Could you check a few things on this model? Use its own coordinates, in mm. A direction names the side the tool comes from. Give positions to 0.01 mm unless a question says otherwise; leave off trailing zeros. Order: outer loops, then holes, each group sorted by start corner. A loop starts at its lowest first (then second) coordinate and runs counter-clockwise, first axis right, second up. Notation, with made-up numbers: (20, 73) - (40, 73) arc R17 cw to (40, 79) - close; hole circle Ø5 at (-18, 41.5). An arc over 180 degrees is marked (long way). Put each result on its own line as item: value.
from build123d import *

# Parameters (mm, degrees)
EXTRUDE_1_DEPTH              = 10
SKETCH_2_3_W                 = 10
SKETCH_2_3_H                 = 57
EXTRUDE_2_DEPTH              = 80
HOLE_WIZARD_M3_2_D           = 3.4
HOLE_WIZARD_M3_2_CSINK_D     = 3.65
HOLE_WIZARD_M3_2_CSINK_ANGLE = 90
CUT_EXTRUDE_1_REACH          = 102.372
HOLE_WIZARD_M3_3_D           = 3.4
HOLE_WIZARD_M3_3_CSINK_D     = 3.65
HOLE_WIZARD_M3_3_CSINK_ANGLE = 90
CHAMFER_2_SIZE               = 3
CHAMFER_3_SIZE               = 6
PATTERN_CIRCULAR_1_COUNT     = 4
SKETCH_13_R                  = 2.5
EXTRUDE_3_DEPTH              = 6
HOLE_WIZARD_M3_1_D           = 2.5
HOLE_WIZARD_M3_1_DEPTH       = 5
HOLE_WIZARD_M3_1_CSINK_D     = 3.05
HOLE_WIZARD_M3_1_CSINK_ANGLE = 90
HOLE_WIZARD_M3_1_TIP         = 0.751075774


with BuildPart() as part:
    # 草图2 → 凸台-拉伸1 (new body)
    with BuildSketch(Plane(origin=(0, 0, 0), x_dir=(1, 0, 0), z_dir=(0, 1, 0))):
        with BuildLine():
            Line((25, 28.5), (0, 28.5))
            ThreePointArc((0, 28.5), (-28.5, 0), (0, -28.5))
            Line((0, -28.5), (25, -28.5))
            Line((25, -28.5), (25, 28.5))
        make_face()
    extrude(amount=EXTRUDE_1_DEPTH)

    # 草图2<3> → 凸台-拉伸2 (add)
    with BuildSketch(Plane(origin=(0, 0, 0), x_dir=(1, 0, 0), z_dir=(0, 1, 0))):
        with Locations((30, 0)):
            Rectangle(SKETCH_2_3_W, SKETCH_2_3_H)
    extrude(amount=EXTRUDE_2_DEPTH)

    # M3 间隙孔2 (through all)
    with Locations(Plane(origin=(0, 10, 0), x_dir=(1, 0, 0), z_dir=(0, 1, 0))):
        with Locations((-13.435028843, 13.435028843), (13.435028843, 13.435028843), (13.435028843, -13.435028843), (-13.435028843, -13.435028843)):
            CounterSinkHole(HOLE_WIZARD_M3_2_D / 2, HOLE_WIZARD_M3_2_CSINK_D / 2, counter_sink_angle=HOLE_WIZARD_M3_2_CSINK_ANGLE)

    # 草图10 → 切除-拉伸1 (cut, up to next)
    with BuildSketch(Plane.ZY.offset(-25), mode=Mode.PRIVATE) as cut_extrude_1_sk1:
        with BuildLine():
            ThreePointArc((-28.5, 51.5), (-20.152543264, 71.652543264), (0, 80))
            Line((0, 80), (-28.5, 80))
            Line((-28.5, 80), (-28.5, 51.5))
        make_face()
    cut_extrude_1_tool1 = extrude(cut_extrude_1_sk1.sketch, amount=-CUT_EXTRUDE_1_REACH, mode=Mode.PRIVATE) & part.part
    # 草图10 → 切除-拉伸1 (cut, up to next)
    with BuildSketch(Plane.ZY.offset(-25), mode=Mode.PRIVATE) as cut_extrude_1_sk2:
        with BuildLine():
            Line((28.5, 80), (0, 80))
            ThreePointArc((0, 80), (20.152543264, 71.652543264), (28.5, 51.5))
            Line((28.5, 51.5), (28.5, 80))
        make_face()
    cut_extrude_1_tool2 = extrude(cut_extrude_1_sk2.sketch, amount=-CUT_EXTRUDE_1_REACH, mode=Mode.PRIVATE) & part.part
    add(cut_extrude_1_tool1.solids().sort_by_distance((25, 73.634014, -22.134014))[0], mode=Mode.SUBTRACT)
    add(cut_extrude_1_tool2.solids().sort_by_distance((25, 73.634014, 22.134014))[0], mode=Mode.SUBTRACT)

    # M3 间隙孔3 (through all)
    with Locations(Plane.ZY.offset(-25)):
        with Locations((13.435028843, 64.935028843)):
            hole_wizard_m3_3 = CounterSinkHole(HOLE_WIZARD_M3_3_D / 2, HOLE_WIZARD_M3_3_CSINK_D / 2, counter_sink_angle=HOLE_WIZARD_M3_3_CSINK_ANGLE)

    # 倒角2
    chamfer_2_edges = [part.edges().sort_by_distance(p)[0] for p in [
        (35, 0, 0),
    ]]
    chamfer(chamfer_2_edges, length=CHAMFER_2_SIZE)

    # 倒角3
    chamfer_3_edges = [part.edges().sort_by_distance(p)[0] for p in [
        (25, 10, 0),
    ]]
    chamfer(chamfer_3_edges, length=CHAMFER_3_SIZE)

    # 阵列(圆周)1: M3 间隙孔3 ×4 about axis
    pattern_circular_1_axis = Axis((0, 51.5, 0), (1, 0, 0))
    for i in range(1, PATTERN_CIRCULAR_1_COUNT):
        add(hole_wizard_m3_3.rotate(pattern_circular_1_axis, i * 360 / PATTERN_CIRCULAR_1_COUNT), mode=Mode.SUBTRACT)

    # 草图13 → 凸台-拉伸3 (add)
    with BuildSketch(Plane(origin=(35, 0, 0), x_dir=(0, 0, -1), z_dir=(1, 0, 0))):
        with Locations((-17.891714588, 56.557050395)):
            Circle(SKETCH_13_R)
        with Locations((18.108285412, 56.557050395)):
            Circle(SKETCH_13_R)
        with Locations((18.108285412, 20.557050395)):
            Circle(SKETCH_13_R)
        with Locations((-17.891714588, 20.557050395)):
            Circle(SKETCH_13_R)
    extrude(amount=EXTRUDE_3_DEPTH)

    # M3 螺纹孔1
    with Locations(Plane(origin=(41, 0, 0), x_dir=(0, 0, -1), z_dir=(1, 0, 0))):
        with Locations((-17.891714588, 56.557050395), (18.108285412, 56.557050395), (-17.891714588, 20.557050395), (18.108285412, 20.557050395)):
            CounterSinkHole(HOLE_WIZARD_M3_1_D / 2, HOLE_WIZARD_M3_1_CSINK_D / 2, depth=HOLE_WIZARD_M3_1_DEPTH, counter_sink_angle=HOLE_WIZARD_M3_1_CSINK_ANGLE)
            with Locations((0, 0, -(HOLE_WIZARD_M3_1_DEPTH + HOLE_WIZARD_M3_1_TIP / 2))):  # 118° drill point
                Cone(0, HOLE_WIZARD_M3_1_D / 2, HOLE_WIZARD_M3_1_TIP, mode=Mode.SUBTRACT)


solid = part.part
1) Suppose I cut it at B-B, the plane y = 13.5. List the corners of the cut face in (x, z) for me.
Filled in:
outline: (22.5, -28.5) - (35, -28.5) - (35, 28.5) - (22.5, 28.5) - close
2) We'd pull the mould along Z, two halves only. Please class faces 4 (the cylindrical face through (37.958, 58.665, -19.452)), 5 (the flat face through (41, 55, 19)): pulls with the +Z half, pulls with the -Z half, needs draft (parallel to the pull), parting line crosses it, or undercut.
Filled in:
face 4: undercut
face 5: needs draft
3) Suppose I cut it at A-A, the plane z = 5. List the corners of the cut face in (x, y) for me, and give its area (3 significant figures).
Filled in:
outline: (-28.06, 0) - (32, 0) - (35, 3) - (35, 79.56) - (25, 79.56) - (25, 16) - (19, 10) - (-28.06, 10) - close
area: 1,340 mm^2
4) I'm going to push flat-ended pins straight in: pin 1 (2 mm diameter, centred on y = 59.5, z = -8.5, fed in from -X); pin 2 (2.5 mm diameter, centred on x = 13.44, z = 13.44, fed in from +Y); pin 3 (24 mm diameter, centred on x = -14.5, z = 9.5, fed in from +Y); pin 4 (1.5 mm diameter, centred on y = 20.56, z = -18.11, fed in from +X). Where does each tip first touch, or does it pass through?
Filled in:
pin 1: stops at x = 25
pin 2: passes through
pin 3: stops at y = 10
pin 4: stops at x = 35.7
5) If I drill on line 1 (Y direction, x = -12, z = -17.5); line 2 (X direction, y = 41.5, z = 11); line 3 (X direction, y = 14, z = 25), over which ranges is the centre line in solid material (lowest first)? Write a range as [from, to].
Filled in:
line 1: y = [0, 10]
line 2: x = [25, 35]
line 3: x = [23, 35]
6) Which directions (+Z, -Z, +X, -X, +Y, -Y) give clear straight access to the entire face, cutting with the end or side of a thin tool? Please do faces 1 (the cylindrical face through (37.958, 58.665, 16.548)), 2 (the flat face through (0, 10, 0)), 3 (the cylindrical face through (30.13, 36.81, 14.58)).
Filled in:
face 1: +X
face 2: +Z, -Z, -X, +Y
face 3: +X, -X
7) Suppose I cut it at C-C, the plane x = 21.5. List the corners of the cut face in (y, z) for me.
Filled in:
outline: (0, -28.5) - (12.5, -28.5) - (12.5, 28.5) - (0, 28.5) - close
8) Suppose I cut it at D-D, the plane x = 14. State how many separate pieces and enclosed holes the cut face has, and give its area (3 significant figures).
Filled in:
separate pieces: 3
enclosed holes: 0
area: 506 mm^2
